from build123d import *

# Parameters (mm, degrees)
SKETCH1_R                       = 17.5
SKETCH1_R_2                     = 7.5
BOSS_EXTRUDE1_DEPTH             = 11
SKETCH1_3_W                     = 75
SKETCH1_3_H                     = 10
BOSS_EXTRUDE2_DEPTH             = 59
TAP_DRILL_FOR_M3X0_5_TAP1_D     = 2.5
TAP_DRILL_FOR_M3X0_5_TAP1_DEPTH = 8
TAP_DRILL_FOR_M3X0_5_TAP1_TIP   = 0.751075774


with BuildPart() as part:
    # Sketch1 → Boss-Extrude1 (new body)
    # profile 1 of 2: a face of its own
    with BuildSketch(Plane.XY):
        with BuildLine():
            Line((37.5, 30), (-37.5, 30))
            Line((-37.5, 30), (-15.160146889, -8.741850278))
            ThreePointArc((-15.160146889, -8.741850278), (-4.524788914, 16.904918967), (17.5, 0))
            ThreePointArc((17.5, 0), (16.904918967, -4.524788914), (15.160146889, -8.741850278))
            Line((15.160146889, -8.741850278), (37.5, 30))
        make_face()
    # profile 2 of 2: a face of its own
    with BuildSketch(Plane.XY):
        Circle(SKETCH1_R)
        Circle(SKETCH1_R_2, mode=Mode.SUBTRACT)
    boss_extrude1 = extrude(amount=-BOSS_EXTRUDE1_DEPTH)

    # Sketch1_3 → Boss-Extrude2 (add)
    with BuildSketch(Plane.XY):
        with Locations((0, 35)):
            Rectangle(SKETCH1_3_W, SKETCH1_3_H)
    extrude(amount=-BOSS_EXTRUDE2_DEPTH)

    # Mirror2: Boss-Extrude1 across plane
    add(boss_extrude1.mirror(Plane.XY.offset(-29.5)))

    # Tap Drill for M3x0.5 Tap1
    with Locations(Plane(origin=(0, 40, 0), x_dir=(1, 0, 0), z_dir=(0, 1, 0))):
        with Locations((-22.5, 53), (22.5, 53), (-24.5, 3.13), (24.5, 3.13)):
            Hole(TAP_DRILL_FOR_M3X0_5_TAP1_D / 2, depth=TAP_DRILL_FOR_M3X0_5_TAP1_DEPTH)
            with Locations((0, 0, -(TAP_DRILL_FOR_M3X0_5_TAP1_DEPTH + TAP_DRILL_FOR_M3X0_5_TAP1_TIP / 2))):  # 118° drill point
                Cone(0, TAP_DRILL_FOR_M3X0_5_TAP1_D / 2, TAP_DRILL_FOR_M3X0_5_TAP1_TIP, mode=Mode.SUBTRACT)


solid = part.part
Model file for the job. Use its own axes, mm. A direction names the side the tool comes from. Give positions to 0.01 mm unless a question says otherwise; leave off trailing zeros. Write each loop counter-clockwise with the first axis right and the second up, starting at its lowest first coordinate (ties: lowest second). Pieces come first, ordered by that corner, then holes. Notation, with made-up numbers: (-8.75, -14) -> (-1.75, -14) arc R29 cw to (-1.75, 15) -> close; hole circle Ø9 at (-29.5, 73). An arc over 180 degrees is marked (long way). Write item = value, one per line.
(1) Mould opens along Y. For faces 4 (the face through (-7.493, 0.33, -5.423)), 5 (the face through (-0.26, -17.5, -53.58)), 6 (the face through (-1, 18, -59)) say: released by +Y, released by -Y, zero draft, split by the parting line, or undercut.
Determined:
face_4 = undercut
face_5 = released by -Y
face_6 = zero draft
(2) Slice it at A-A, the plane y = 12. Give the cut face in (x, z).
Determined:
outline = (-27.12, -59) -> (27.12, -59) -> (27.12, -48) -> (-27.12, -48) -> close; (-27.12, -11) -> (27.12, -11) -> (27.12, 0) -> (-27.12, 0) -> close
(3) Probe line 1 along X through (y, z) = (37, -3); line 2 along X through (y, z) = (34.75, -53); line 3 along Z through (x, y) = (-8.5, 26). List the from-to ranges inside material, lowest first.
Determined:
line_1 = -37.5 to -25.74, -23.26 to 23.26, 25.74 to 37.5
line_2 = -37.5 to -23.75, -21.25 to 21.25, 23.75 to 37.5
line_3 = -59 to -48, -11 to 0
(4) Slice it at C-C, the plane y = 1. Give the cut face in (x, z).
Determined:
outline = (-20.78, -59) -> (-7.43, -59) -> (-7.43, -48) -> (-20.78, -48) -> close; (-20.78, -11) -> (-7.43, -11) -> (-7.43, 0) -> (-20.78, 0) -> close; (7.43, -59) -> (20.78, -59) -> (20.78, -48) -> (7.43, -48) -> close; (7.43, -11) -> (20.78, -11) -> (20.78, 0) -> (7.43, 0) -> close
(5) Slice it at D-D, the plane x = 18. Give the cut face in (y, z), then the cut area to 3 significant figures.
Determined:
outline = (-3.82, -59) -> (40, -59) -> (40, 0) -> (-3.82, 0) -> (-3.82, -11) -> (30, -11) -> (30, -48) -> (-3.82, -48) -> close
area = 1,330 mm2
(6) Tool access for faces 1 (the face through (-22.34, 35.94, -54.24)), 2 (the face through (-1, 30, -29)), 3 (the face through (26.2, 10.4, -5.4)): list every direction of +Z, -Z, +X, -X, +Y, -Y with a clear straight run to the whole face (end or side of a thin tool).
Determined:
face_1 = +Y
face_2 = +X, -X, -Y
face_3 = +Z, -Z, +X, -Y
(7) Flat gauge pins, fed straight in: P1, Ø2, axis at x = -24.5, z = -3.13, coming from the +Y side; P2, Ø1.5, axis at x = -7.5, z = -27, coming from the -Y side; P3, Ø4, axis at x = 24.5, z = -3.13, coming from the -Y side. Where does each tip first touch, or does it go through?
Determined:
P1 = 31.85
P2 = 30
P3 = 3.99
(8) Slice it at B-B, the plane x = 5. Give the cut face in (y, z), then the cut area to 3 significant figures.
Determined:
outline = (-16.77, -59) -> (-5.59, -59) -> (-5.59, -48) -> (-16.77, -48) -> close; (-16.77, -11) -> (-5.59, -11) -> (-5.59, 0) -> (-16.77, 0) -> close; (5.59, -59) -> (40, -59) -> (40, 0) -> (5.59, 0) -> (5.59, -11) -> (30, -11) -> (30, -48) -> (5.59, -48) -> close
area = 1,370 mm2
